Build history of the part. All positions in model axes, mm. A direction names the side the tool comes from. Give positions to 0.01 mm unless a question says otherwise; leave off trailing zeros. Order: outer loops, then holes, each group sorted by start corner. A loop starts at its lowest first (then second) coordinate and runs counter-clockwise, first axis right, second up. Notation, with made-up numbers: M 58.25,-30 L 97.25,-30 A13 ccw 97.25,-24 Z; hole C 13.25,-23.5 d2. An arc over 180 degrees is marked long. One line per item, written item: value. Start each with the question number.
from build123d import *

# Parameters (mm, degrees)
ESQUISSE3_W             = 155
ESQUISSE3_H             = 125
BOSS_EXTRU_1_DEPTH      = 50
ESQUISSE4_W             = 145
ESQUISSE4_H             = 115
ENL_V_MAT_EXTRU_1_DEPTH = 45
CONG_1_R                = 5


with BuildPart() as part:
    # Esquisse3 → Boss.-Extru.1 (new body)
    with BuildSketch(Plane(origin=(0, 0, 0), x_dir=(1, 0, 0), z_dir=(0, 1, 0))):
        Rectangle(ESQUISSE3_W, ESQUISSE3_H)
    extrude(amount=BOSS_EXTRU_1_DEPTH)

    # Esquisse4 → Enlèv. mat.-Extru.1 (cut)
    with BuildSketch(Plane(origin=(0, 50, 0), x_dir=(1, 0, 0), z_dir=(0, 1, 0))):
        Rectangle(ESQUISSE4_W, ESQUISSE4_H)
    extrude(amount=-ENL_V_MAT_EXTRU_1_DEPTH, mode=Mode.SUBTRACT)

    # Congé1
    cong_1_edges = [part.edges().sort_by_distance(p)[0] for p in [
        (0, 0, -62.5),
        (77.5, 0, 0),
        (0, 0, 62.5),
        (-77.5, 0, 0),
        (-77.5, 25, -62.5),
        (77.5, 25, -62.5),
        (77.5, 25, 62.5),
        (-77.5, 25, 62.5),
    ]]
    fillet(cong_1_edges, radius=CONG_1_R)


solid = part.part
1) Tool access for faces 4 (the flat face through (-1, 5, -1)), 5 (the flat face through (-1, 0, -1)): list every direction of +Z, -Z, +X, -X, +Y, -Y with a clear straight run to the whole face (end or side of a thin tool).
2) Pull direction X, two halves, no side cores. Call faces 1 (the cylindrical face through (76, 1.43, -0.8)), 2 (the flat face through (-72.5, 28, 1)), 3 (the cylindrical face through (-76.07, 27.82, -61)): pulls with the +X half, pulls with the -X half, needs draft (parallel to the pull), parting line crosses it, or undercut.
3) Drill centre lines: line 1 (X direction, y = 48.5, z = -46); line 2 (Z direction, x = 62.5, y = 9.5); line 3 (Y direction, x = -63, z = 49.5). Where is each one in solid material? Low to high.
4) Drop a flat-ended pin along its axis: P1, Ø4, axis at x = 25, z = 36.5, coming from the +Y side. Give the stop position or say it passes through.
5) Slice it at B-B (x = 14). List the corners of the cut face in (y, z).
6) Slice it at C-C (z = 49). List the corners of the cut face in (x, y), plus the area to 3 significant figures.
7) Slice it at A-A (y = 34). List the corners of the cut face in (x, z), plus the area to 3 significant figures.
Results list:
1. face 4: +Y
1. face 5: +Z, -Z, +X, -X, -Y
2. face 1: pulls with the +X half
2. face 2: undercut
2. face 3: pulls with the -X half
3. line 1: x = -77.5 to -72.5, 72.5 to 77.5
3. line 2: z = -62.5 to -57.5, 57.5 to 62.5
3. line 3: y = 0 to 5
4. P1: stops at y = 5
5. outline: M 0,-57.5 A5 ccw 5,-62.5 L 50,-62.5 L 50,-57.5 L 5,-57.5 L 5,57.5 L 50,57.5 L 50,62.5 L 5,62.5 A5 ccw 0,57.5 Z
6. outline: M -77.5,5 A5 ccw -72.5,0 L 72.5,0 A5 ccw 77.5,5 L 77.5,50 L 72.5,50 L 72.5,5 L -72.5,5 L -72.5,50 L -77.5,50 Z
6. area: 1,210 mm²
7. outline: M -77.5,-57.5 A5 ccw -72.5,-62.5 L 72.5,-62.5 A5 ccw 77.5,-57.5 L 77.5,57.5 A5 ccw 72.5,62.5 L -72.5,62.5 A5 ccw -77.5,57.5 Z; hole M -72.5,-57.5 L 72.5,-57.5 L 72.5,57.5 L -72.5,57.5 Z
7. area: 2,680 mm²
